from build123d import *

# Parameters (mm, degrees)
SKETCH1_W               = 34
SKETCH1_H               = 16
BOSS_EXTRUDE1_DEPTH     = 2
CUT_EXTRUDE1_DEPTH      = 19.894443628
CUT_EXTRUDE1_DEPTH_BACK = 19.894443628
SKETCH2_W               = 23
SKETCH2_H               = 12
SKETCH3_R               = 0.8
CUT_EXTRUDE5_DEPTH      = 2


with BuildPart() as part:
    # Sketch1 → Boss-Extrude1 (new body)
    with BuildSketch(Plane(origin=(0, 0, 0), x_dir=(1, 0, 0), z_dir=(0, 1, 0))):
        Rectangle(SKETCH1_W, SKETCH1_H)
    extrude(amount=BOSS_EXTRUDE1_DEPTH)

    # Sketch2 → Cut-Extrude1 (cut, two sides: drawn at the far end of the back side and taken through both)
    with BuildSketch(Plane(origin=(0, 2, 0), x_dir=(1, 0, 0), z_dir=(0, 1, 0)).offset(-CUT_EXTRUDE1_DEPTH_BACK)):
        with Locations((-0.5, 0)):
            Rectangle(SKETCH2_W, SKETCH2_H)
    extrude(amount=CUT_EXTRUDE1_DEPTH + CUT_EXTRUDE1_DEPTH_BACK, mode=Mode.SUBTRACT)

    # Sketch3 → Cut-Extrude5 (cut)
    with BuildSketch(Plane(origin=(0, 0, 0), x_dir=(1, 0, 0), z_dir=(0, 1, 0))):
        with Locations(Location((-14.5, 0, 0), (0, 0, 270))):
            Circle(SKETCH3_R)
        with Locations(Location((13, 0, 0), (0, 0, 270))):
            Circle(SKETCH3_R)
    extrude(amount=CUT_EXTRUDE5_DEPTH, mode=Mode.SUBTRACT)


solid = part.part
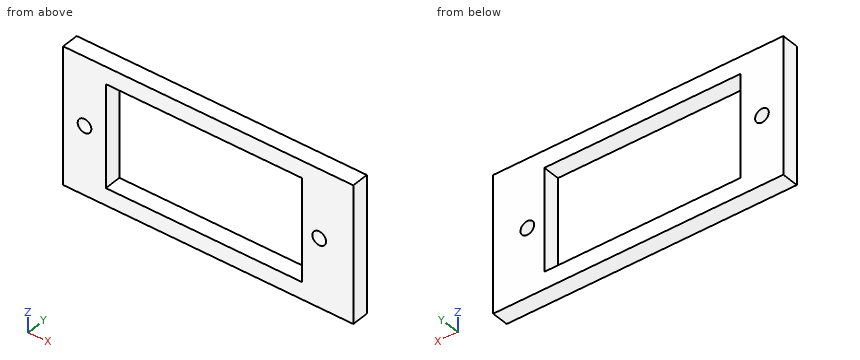
Verification items for the finished model (mm, model axes). Round coordinates to 2 decimals unless told otherwise and drop trailing zeros. Loops run counter-clockwise (first coordinate to the right, second up) from the corner with the lowest first, then second, coordinate; pieces in that order, holes last. Notation, with made-up numbers: (68.5, -8) - (114.5, -8) arc R30 cw to (114.5, 23) - close; hole circle Ø1 at (-11, 38). An arc over 180 degrees is marked (long way). Use a Markdown table: item, result. Add a question column.
1. Section check A-A, the plane z = 1.25. Record the boundary of the cut face in (x, y), plus the area to 3 significant figures.
2. Gauge pin test, flat end, axial feed: pin 1 (2 mm diameter, centred on x = -14.5, z = 0, fed in from -Y). Record the tip position at first contact, or that the pin passes through.
3. Section check B-B, the plane x = 13. Record the boundary of the cut face in (y, z), plus the area to 3 significant figures.
4. Section check C-C, the plane y = 1.3. Record the boundary of the cut face in (x, z).
5. Thickness scan on probe 1 along X at (y, z) = (1.2, 0); probe 2 along Z at (x, y) = (5, 0.5); probe 3 along X at (y, z) = (0.65, -1.75). Record the ranges inside material, lowest first. Write a range as [from, to].
Checks:
| question | item | result |
|---|---|---|
| 1 | outline | (-17, 0) - (-12, 0) - (-12, 2) - (-17, 2) - close; (11, 0) - (17, 0) - (17, 2) - (11, 2) - close |
| 1 | area | 22.0 mm^2 |
| 2 | pin 1 | stops at y = 0 |
| 3 | outline | (0, -8) - (2, -8) - (2, -0.8) - (0, -0.8) - close; (0, 0.8) - (2, 0.8) - (2, 8) - (0, 8) - close |
| 3 | area | 28.8 mm^2 |
| 4 | outline | (-17, -8) - (17, -8) - (17, 8) - (-17, 8) - close; hole circle Ø1.6 at (-14.5, 0); hole (-12, -6) - (11, -6) - (11, 6) - (-12, 6) - close; hole circle Ø1.6 at (13, 0) |
| 5 | probe 1 | x = [-17, -15.3], [-13.7, -12], [11, 12.2], [13.8, 17] |
| 5 | probe 2 | z = [-8, -6], [6, 8] |
| 5 | probe 3 | x = [-17, -12], [11, 17] |
